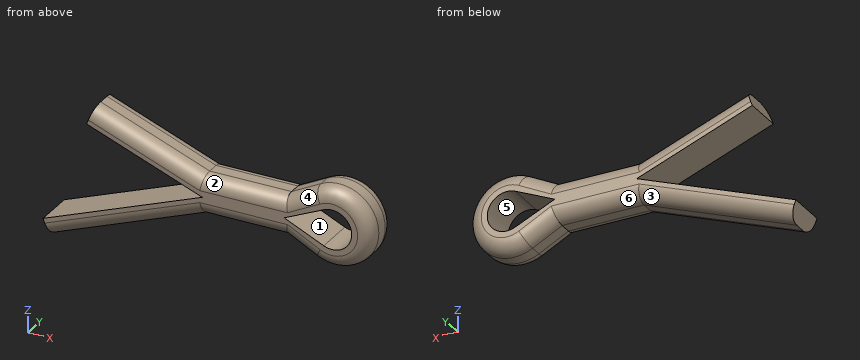
Autodesk Inventor part; units mm, degrees
ref_plane "Work Plane1" through (0, -10, 0) normal (0, 0, -1) x (0, 1, 0)
ref_plane "Work Plane3" through (0, 0, 1.45) normal (-1, 0, 0) x (0, 1, 0)
ref_plane "YZ Plane" through (0, 0, 0) normal (1, 0, 0) x (0, 1, 0)
sketch "Skizze1" plane through (0, 0, 0) normal (0, 1, 0) x (-1, 0, 0)
  arc A0 (-2.1633, 2.5736) -> (-2.1633, -2.5736) centre (-3.5, 0) ccw
  arc A1 (-2.8993, 1.3197) -> (-2.8993, -1.3197) centre (-3.5, 0) ccw
  line L0 (0, 1.45) -> (6, 1.45)
  line L1 (0, -1.45) -> (6, -1.45)
  line L2 (6, 1.45) -> (14, 4.515)
  line L3 (14, 4.515) -> (14.4844, 3.2505)
  line L4 (14.4844, 3.2505) -> (6, 0)
  line L5 (6, 0) -> (17.6844, -4.4765)
  line L6 (17.6844, -4.4765) -> (17.2, -5.7409)
  line L7 (17.2, -5.7409) -> (6, -1.45)
  line L8 (0, 0) -> (-2.8993, -1.3197)
  line L9 (0, 0) -> (-2.8993, 1.3197)
  line L10 (0, 1.45) -> (0, -1.45) construction
  line L11 (0, 1.45) -> (-2.1633, 2.5736)
  line L12 (0, -1.45) -> (-2.1633, -2.5736)
  line L13 (-6.4, 0) -> (6, 0) construction
  line L14 (6, 1.45) -> (6, -1.45) construction
  dimension "d0" = 6
  dimension "d1" = 14
  dimension "d2" = 159.037
  dimension "d3" = 159.037
  dimension "d4" = 3.2
  dimension "d5" = 1.45
  dimension "d6" = 2.9
  dimension "d7" = 1.45
  dimension "d8" = 1.45
  dimension "d9" = 3.5
extrude "Körper" add sketch "Skizze1" along normal mid plane 2.9
fillet "Rundung" radius 1.015 14 edges at (-10, -1.45, 2.9825) (-10, 1.45, 2.9825) (-3, -1.45, 1.45) (-3, 1.45, 1.45) (6.4, -1.45, 0) (1.0817, -1.45, -2.0118) (1.0817, -1.45, 2.0118) (6.4, 1.45, 0) (1.0817, 1.45, 2.0118) (1.0817, 1.45, -2.0118) (-3, -1.45, -1.45) (-11.6, -1.45, -3.5955) (-3, 1.45, -1.45) (-11.6, 1.45, -3.5955)
ref_plane "Work Plane1" through (0, -10, 0) normal (0, 0, -1) x (0, 1, 0)
ref_plane "Work Plane3" through (0, 0, 1.45) normal (-1, 0, 0) x (0, 1, 0)
equation "\"d0\" = MSIAB"
equation "\"d1\" = SNLG"
equation "\"d4\" = LGDIF"
equation "\"d5\" = -0.5 * SNND1 + 0.5 * KBR"
equation "\"d6\" = 0.5 * KBR"
equation "\"d7\" = 0.5 * SNND1"
equation "\"d8\" = 0.5 * SNND1"
equation "\"d9\" = KOL - 0.5 * KBR"
equation "\"d10\" = SNND1"
equation "\"d12\" = 0.35 * SNND1"
equation "\"SNND\" = 3.2"
equation "\"SNLG\" = 14"
equation "\"SNND1\" = 2.9"
equation "\"KBR\" = 5.8"
equation "\"KOL\" = 6.4"
equation "\"LGDIF\" = 3.2"
equation "\"MSIAB\" = 6"
equation "\"NNDMAX\" = 14"
equation "\"DSH\" = 6"
equation "\"NNDMIN\" = 11"
properties part number "ISO 1234 - 3,2 x 14" material "Stahl"
The listing builds one solid part. Answer for the finished solid, in the listing's coordinates (mm). Face numbers are marked on the shaded views. A direction names the side the tool comes from. Give positions to 0.01 mm unless a question says otherwise; leave off trailing zeros. Order: outer loops, then holes, each group sorted by start corner. A loop starts at its lowest first (then second) coordinate and runs counter-clockwise, first axis right, second up.
Item 1: Find the intervals of material crossed by probe 1 along Z at (x, y) = (3.5, 0.3); probe 2 along Z at (x, y) = (-10.75, 1.15); probe 3 along Y at (x, z) = (-2.75, -0.5), in increasing order.
From the geometry:
probe 1: z = -2.9 to -1.45, 1.45 to 2.9
probe 2: z = -2.95 to -1.82, 1.82 to 2.95
probe 3: y = -1.45 to 1.45
Item 2: The part is cut by section C-C, the plane y = -1.1. Give the vertices of the cut face in (x, z).
From the geometry:
outline: (-17.68, -4.48) - (-17.29, -5.51) - (-6.05, -1.2) - (0.06, -1.2) - (2.28, -2.35) arc R2.65 ccw (long way) to (2.28, 2.35) - (0.06, 1.2) - (-6.05, 1.2) - (-14.09, 4.28) - (-14.48, 3.25) - (-6, 0) - close; hole (0, 0) - (2.9, -1.32) arc R1.45 ccw (long way) to (2.9, 1.32) - close
Item 3: Given pin 1 Ø5 at (x, z) = (-2, -1.5) entering from +Y; pin 2 Ø2 at (x, z) = (-5.5, -4) entering from -Y, each flat-ended and moving along its own axis, determine where each tip first touches the part or whether it passes through.
From the geometry:
pin 1: stops at y = 1.45
pin 2: passes through
Item 4: The part is cut by section B-B, the plane x = 3.5. Give the vertices of the cut face in (y, z) (3 decimals), and give its area (3 significant figures).
From the geometry:
outline: (-1.45, -1.885) arc R1.015 ccw to (-0.435, -2.9) - (0.435, -2.9) arc R1.015 ccw to (1.45, -1.885) - (1.45, -1.45) - (-1.45, -1.45) - close; (-1.45, 1.45) - (1.45, 1.45) - (1.45, 1.885) arc R1.015 ccw to (0.435, 2.9) - (-0.435, 2.9) arc R1.015 ccw to (-1.45, 1.885) - close
area: 7.53 mm2
Item 5: Which of the six approach directions +Z, -Z, +X, -X, +Y, -Y give full straight-line access (tool end or side, diameter ignored) to the marked faces 1, 2 and 3?
From the geometry:
face 1: +Y, -Y
face 2: +Z, -Y
face 3: -Z, +Y
Item 6: For a pull along Z with two mould halves and no side action, classify the marked faces 4, 5 and 6 as pulls with the +Z half, pulls with the -Z half, needs draft (parallel to the pull), parting line crosses it, or undercut.
From the geometry:
face 4: pulls with the +Z half
face 5: undercut
face 6: pulls with the -Z half
